Study the drawing (mm; zero at the part's minimum x, y, z) and answer. A direction names the side the tool comes from. Give positions to 0.01 mm unless a question says otherwise; leave off trailing zeros. Order: outer loops, then holes, each group sorted by start corner. A loop starts at its lowest first (then second) coordinate and runs counter-clockwise, first axis right, second up.
Item 1: A cutting plane is placed at C-C (y = 2.05). Write down the section's boundary in (x, z).
Item 2: Given pin 1 Ø1.6 at (y, z) = (2.5, 16) entering from -X; pin 2 Ø0.5 at (y, z) = (2.5, 16) entering from +X; pin 3 Ø1.5 at (x, y) = (4, 2.5) entering from +Z, each flat-ended and moving along its own axis, determine where each tip first touches the part or whether it passes through.
Item 3: A cutting plane is placed at B-B (y = 4.6). Write down the section's boundary in (x, z).
Item 4: Which of the six approach directions +Z, -Z, +X, -X, +Y, -Y give full straight-line access (tool end or side, diameter ignored) to the marked faces 1 and 2?
Item 5: Find the intervals of material crossed by line 1 along Z through (x, y) = (8.75, 0.95); line 2 along X through (y, z) = (2.1, 15.75); line 3 along Z through (x, y) = (4, 2.95), in increasing order.
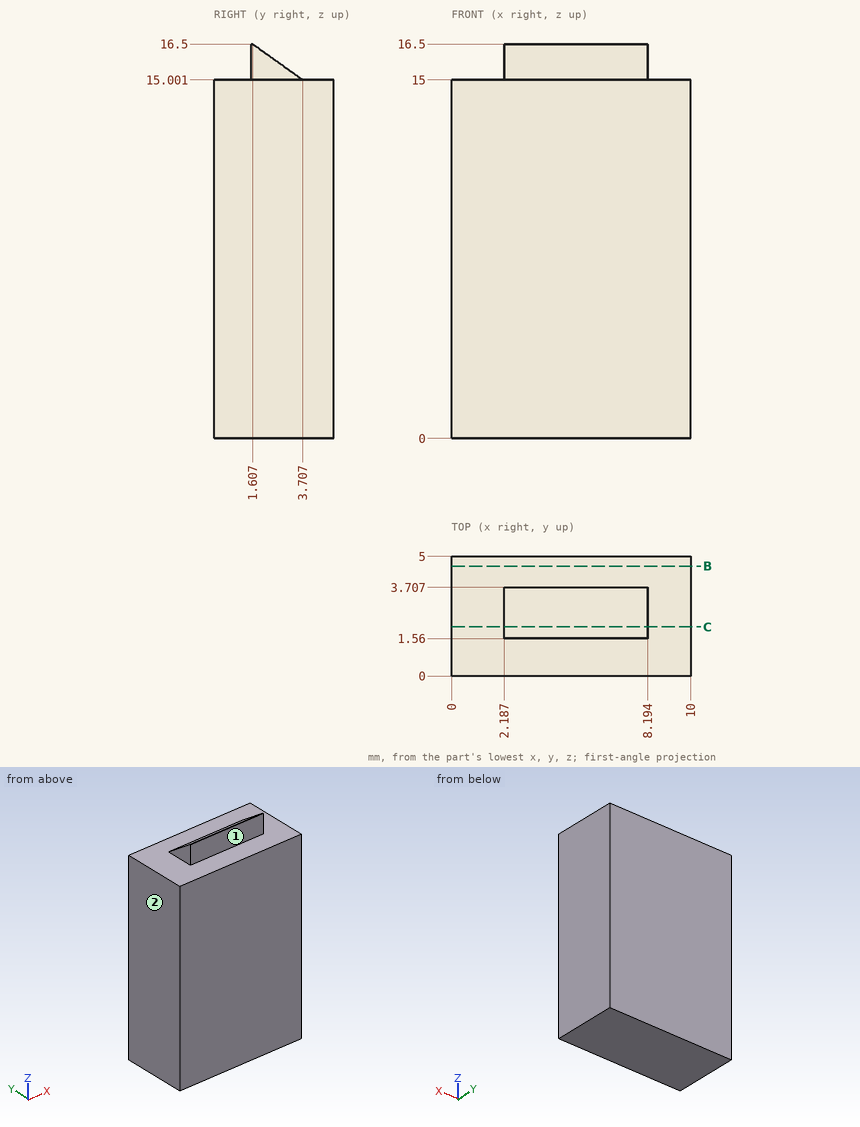
Response values:
1. outline: (0, 0) - (10, 0) - (10, 15) - (8.19, 15) - (8.19, 16.18) - (2.19, 16.18) - (2.19, 15) - (0, 15) - close
2. pin 1: stops at x = 2.19
2. pin 2: stops at x = 8.19
2. pin 3: stops at z = 16.4
3. outline: (0, 0) - (10, 0) - (10, 15) - (0, 15) - close
4. face 1: +Z, +X, -X, -Y
4. face 2: +Z, -Z, -X, +Y, -Y
5. line 1: z = 0 to 15
5. line 2: x = 2.19 to 8.19
5. line 3: z = 0 to 15.54
